For this review, take the finished solid that the model builds, in its own axes (mm). A direction names the side the tool comes from. Coordinates: 2 decimals unless noted, no trailing zeros. Write each loop counter-clockwise with the first axis right and the second up, starting at its lowest first coordinate (ties: lowest second). Pieces come first, ordered by that corner, then holes. Notation, with made-up numbers: (39.25, 29.5) -> (54.25, 29.5) arc R22 ccw to (54.25, 64.5) -> close; hole circle Ø3 at (1.25, 76). An arc over 180 degrees is marked (long way). One line per item, written item: value. Start each with the question number.
1) Add section A-A (x = 40.5). State the section outline as (y, z) points.
2) For probe 1 along X at (y, z) = (-0.8, -5); probe 2 along X at (y, z) = (0.9, 41); probe 3 along Z at (x, y) = (34, -0.25), list the stretches that pass through material, from the lowest coordinate up. Write a range as from..to.
3) Machinability: for faces 1 (the cylindrical face through (-37.255, 0.515, 43.594)), 2 (the cylindrical face through (-52.28, 0.52, -39.67)), 3 (the flat face through (8, 0, 34)), 4 (the cylindrical face through (-52.2, 0.52, -28.41)), which of the approach directions +Z, -Z, +X, -X, +Y, -Y give a long, thin tool a straight path to every point of the face, cutting with its end or side? Answer none if there is none.
4) Add section B-B (z = -31.5). State the section outline as (x, y) points.
5) Add section D-D (x = -48). State the section outline as (y, z) points, and give its area (3 significant figures).
6) Mouldability with a two-part tool opening along Z and no side actions: class faces 5 (the flat face through (51, 1.016, -34)), 6 (the cylindrical face through (52.351, 0.515, 28.634)), 7 (the cylindrical face through (-52.24, 0.52, 43.55)) as released by +Z, released by -Z, zero draft, split by the parting line, or undercut.
7) For pin 1 Ø0.8 at (y, z) = (0.5, 35.5) entering from -X; pin 2 Ø0.5 at (y, z) = (0.5, -32.5) entering from +X; pin 3 Ø0.5 at (x, y) = (42, 0.5) entering from -Z, all flat-tipped, find the tip position at first contact; note any pin that passes through.
8) Add section C-C (y = -0.35). State the section outline as (x, z) points.
from build123d import *

# Parameters (mm, degrees)
SKETCH2_W            = 3.747831998
SKETCH2_H            = 12.799678195
SKETCH2_H_2          = 12.611039135
SKETCH2_W_2          = 3.862926877
BOSS_EXTRUDE2_DEPTH  = 1.016
SKETCH2_7_W          = 112.7125
SKETCH2_7_H          = 93.6625
BOSS_EXTRUDE14_DEPTH = 1.27
SKETCH2_8_W          = 89.425
SKETCH2_8_H          = 67.9625
CUT_EXTRUDE4_DEPTH   = 1.27
FILLET5_R            = 2.54
FILLET6_R            = 2.54
FILLET7_R            = 2.54
FILLET8_R            = 2.54
FILLET9_R            = 1.27
FILLET10_R           = 1.27
FILLET11_R           = 1.27
FILLET12_R           = 1.27


with BuildPart() as part:
    # Sketch2 → Boss-Extrude2 (new body)
    with BuildSketch(Plane(origin=(0, 0, 0), x_dir=(1, 0, 0), z_dir=(0, 1, 0))):
        with Locations((-51.086415999, 34.081410903)):
            Rectangle(SKETCH2_W, SKETCH2_H)
        with Locations((-51.086415999, -34.175730433)):
            Rectangle(SKETCH2_W, SKETCH2_H_2)
        Polygon((-36.491625106, -40.48125), (-49.2125, -40.48125), (-52.960331998, -40.48125), (-52.960331998, -44.318627665), (-36.491625106, -44.318627665), align=None)
        Polygon((49.2125, -40.48125), (36.537927314, -40.48125), (36.537927314, -44.318627665), (53.075426877, -44.318627665), (53.075426877, -40.48125), align=None)
        with Locations((51.143963439, -34.175730433)):
            Rectangle(SKETCH2_W_2, SKETCH2_H_2)
        with Locations((51.143963439, 34.081410903)):
            Rectangle(SKETCH2_W_2, SKETCH2_H)
    extrude(amount=BOSS_EXTRUDE2_DEPTH)

    # Sketch2_7 → Boss-Extrude14 (add)
    with BuildSketch(Plane(origin=(0, 0, 0), x_dir=(1, 0, 0), z_dir=(0, 1, 0))):
        Rectangle(SKETCH2_7_W, SKETCH2_7_H)
    extrude(amount=-BOSS_EXTRUDE14_DEPTH)

    # Sketch2_8 → Cut-Extrude4 (cut)
    with BuildSketch(Plane(origin=(0, 0, 0), x_dir=(1, 0, 0), z_dir=(0, 1, 0))):
        with Locations((-0.5, 2.5)):
            Rectangle(SKETCH2_8_W, SKETCH2_8_H)
    extrude(amount=-CUT_EXTRUDE4_DEPTH, mode=Mode.SUBTRACT)

    # Fillet5
    fillet5_edges = [part.edges().sort_by_distance(p)[0] for p in [
        (-52.960331998, 0.508, -40.48125),
        (-52.960331998, 0.508, -27.681571805),
    ]]
    fillet(fillet5_edges, radius=FILLET5_R)

    # Fillet6
    fillet6_edges = [part.edges().sort_by_distance(p)[0] for p in [
        (53.075426877, 0.508, -27.681571805),
        (53.075426877, 0.508, -40.48125),
    ]]
    fillet(fillet6_edges, radius=FILLET6_R)

    # Fillet7
    fillet7_edges = [part.edges().sort_by_distance(p)[0] for p in [
        (-52.960331998, 0.508, 27.870210865),
        (-52.960331998, 0.508, 44.318627665),
        (-36.491625106, 0.508, 44.318627665),
    ]]
    fillet(fillet7_edges, radius=FILLET7_R)

    # Fillet8
    fillet8_edges = [part.edges().sort_by_distance(p)[0] for p in [
        (36.537927314, 0.508, 44.318627665),
        (53.075426877, 0.508, 44.318627665),
        (53.075426877, 0.508, 27.870210865),
    ]]
    fillet(fillet8_edges, radius=FILLET8_R)

    # Fillet9
    # the kernel refuses this fillet: 1.27 mm, written as the material it adds along each edge
    # the kernel refuses this fillet: 1.27 mm, written as the material it takes off along each edge
    with BuildSketch(Plane(origin=(-49.2125, 0, 27.870210865), x_dir=(-0.9999973876503099, 0, 0.00228575863903478), z_dir=(0, 1, 0))) as fillet9_2_piece_1:
        with BuildLine():
            CenterArc((1.272903076, 1.268616276), FILLET9_R, 179.869035563, 92.8058175)
            Line((0.002906394, 1.27151919), (-0.124093275, 1.271809481))
            Line((-0.124093275, 1.271809481), (-0.126999668, 0.000290291))
            Line((-0.126999668, 0.000290291), (-0.000290291, -0.126999668))
            ThreePointArc((-0.000290291, -0.126999668), (1.207538551, -0.129760481), (1.338098323, -0.126861628))
            Line((1.338098323, -0.126861628), (1.332171482, 0))
        make_face()
    extrude(amount=4.346428706, mode=Mode.SUBTRACT)
    with BuildSketch(Plane(origin=(-46.0375, 1.016, 27.870210865), x_dir=(0, -1, 0), z_dir=(-1, 0, 0))) as fillet9_2_piece_2_section:
        with BuildLine():
            CenterArc((FILLET9_R, FILLET9_R), FILLET9_R, 180, 90)
            Line((0, FILLET9_R), (0, 0))
            Line((0, 0), (FILLET9_R, 0))
        make_face()
    fillet9_2_piece_2 = extrude(amount=4.382831998, mode=Mode.PRIVATE)
    fillet9_2_piece_2 = split(fillet9_2_piece_2, bisect_by=Plane(origin=(-49.536450459, 0, 27.947431498), z_dir=(0, 1, 0)), keep=Keep.TOP, mode=Mode.PRIVATE)
    fillet9_2_piece_2 = fillet9_2_piece_2 - Plane(origin=(-50.420331998, 0.588239607, 30.410210865), x_dir=(0, 0, -1), z_dir=(0, 1, 0)) * Cylinder(2.54, 14, mode=Mode.PRIVATE)
    add(fillet9_2_piece_2, mode=Mode.SUBTRACT)

    # Fillet10
    fillet10_edges = [part.edges().sort_by_distance(p)[0] for p in [
        (-49.2125, 0.508, -40.48125),
    ]]
    fillet(fillet10_edges, radius=FILLET10_R)

    # Fillet11
    fillet11_edges = [part.edges().sort_by_distance(p)[0] for p in [
        (49.2125, 0.508, 27.870210865),
    ]]
    fillet(fillet11_edges, radius=FILLET11_R)

    # Fillet12
    fillet12_edges = [part.edges().sort_by_distance(p)[0] for p in [
        (49.2125, 0.508, -40.48125),
    ]]
    fillet(fillet12_edges, radius=FILLET12_R)


solid = part.part
Numbers:
1. outline: (-1.27, -46.83) -> (0, -46.83) -> (0, -36.48) -> (-1.27, -36.48) -> close; (-1.27, 31.48) -> (0, 31.48) -> (0, 40.48) -> (1.02, 40.48) -> (1.02, 44.32) -> (0, 44.32) -> (0, 46.83) -> (-1.27, 46.83) -> close
2. probe 1: -56.36..-45.21, 44.21..56.36
2. probe 2: -52.96..-36.49, 36.54..53.08
2. probe 3: -46.83..-36.48, 31.48..46.83
3. face 1: +Z, +Y
3. face 2: -Z, -X, +Y
3. face 3: +Y
3. face 4: -X, +Y
4. outline: (-56.36, -1.27) -> (-45.21, -1.27) -> (-45.21, 0) -> (-49.21, 0) -> (-49.21, 1.02) -> (-52.96, 1.02) -> (-52.96, 0) -> (-56.36, 0) -> close; (44.21, -1.27) -> (56.36, -1.27) -> (56.36, 0) -> (53.08, 0) -> (53.08, 1.02) -> (49.21, 1.02) -> (49.21, 0) -> (44.21, 0) -> close
5. outline: (-1.27, -46.83) -> (0, -46.83) -> (0, 40.48) -> (1.02, 40.48) -> (1.02, 44.32) -> (0, 44.32) -> (0, 46.83) -> (-1.27, 46.83) -> close
5. area: 123 mm²
6. face 5: zero draft
6. face 6: undercut
6. face 7: released by +Z
7. pin 1: x = -52.96
7. pin 2: x = 53.08
7. pin 3: z = 40.48
8. outline: (-56.36, -46.83) -> (56.36, -46.83) -> (56.36, 46.83) -> (-56.36, 46.83) -> close; hole (-45.21, -36.48) -> (44.21, -36.48) -> (44.21, 31.48) -> (-45.21, 31.48) -> close
